from build123d import *

# Parameters (mm, degrees)
SKETCH1_R           = 2.5
BOSS_EXTRUDE1_DEPTH = 180


with BuildPart() as part:
    # Sketch1 → Boss-Extrude1 (new body)
    with BuildSketch(Plane.XY):
        with BuildLine():
            Line((2.839339828, 3.9), (5.5, 6.560660172))
            Line((5.5, 6.560660172), (5.5, 8.2))
            Line((5.5, 8.2), (3.1, 8.2))
            Line((3.1, 8.2), (3.1, 9.5))
            Line((3.1, 9.5), (3.6, 9.5))
            Line((3.6, 9.5), (3.6, 10))
            Line((3.6, 10), (8.5, 10))
            ThreePointArc((8.5, 10), (9.560660172, 9.560660172), (10, 8.5))
            Line((10, 8.5), (10, 3.6))
            Line((10, 3.6), (9.5, 3.6))
            Line((9.5, 3.6), (9.5, 3.1))
            Line((9.5, 3.1), (8.2, 3.1))
            Line((8.2, 3.1), (8.2, 5.5))
            Line((8.2, 5.5), (6.560660172, 5.5))
            Line((6.560660172, 5.5), (3.9, 2.839339828))
            Line((3.9, 2.839339828), (3.9, -2.839339828))
            Line((3.9, -2.839339828), (6.560660172, -5.5))
            Line((6.560660172, -5.5), (8.2, -5.5))
            Line((8.2, -5.5), (8.2, -3.1))
            Line((8.2, -3.1), (9.5, -3.1))
            Line((9.5, -3.1), (9.5, -3.6))
            Line((9.5, -3.6), (10, -3.6))
            Line((10, -3.6), (10, -8.5))
            ThreePointArc((10, -8.5), (9.560660172, -9.560660172), (8.5, -10))
            Line((8.5, -10), (3.6, -10))
            Line((3.6, -10), (3.6, -9.5))
            Line((3.6, -9.5), (3.1, -9.5))
            Line((3.1, -9.5), (3.1, -8.2))
            Line((3.1, -8.2), (5.5, -8.2))
            Line((5.5, -8.2), (5.5, -6.560660172))
            Line((5.5, -6.560660172), (2.839339828, -3.9))
            Line((2.839339828, -3.9), (-2.839339828, -3.9))
            Line((-2.839339828, -3.9), (-5.5, -6.560660172))
            Line((-5.5, -6.560660172), (-5.5, -8.2))
            Line((-5.5, -8.2), (-3.1, -8.2))
            Line((-3.1, -8.2), (-3.1, -9.5))
            Line((-3.1, -9.5), (-3.6, -9.5))
            Line((-3.6, -9.5), (-3.6, -10))
            Line((-3.6, -10), (-8.5, -10))
            ThreePointArc((-8.5, -10), (-9.560660172, -9.560660172), (-10, -8.5))
            Line((-10, -8.5), (-10, -3.6))
            Line((-10, -3.6), (-9.5, -3.6))
            Line((-9.5, -3.6), (-9.5, -3.1))
            Line((-9.5, -3.1), (-8.2, -3.1))
            Line((-8.2, -3.1), (-8.2, -5.5))
            Line((-8.2, -5.5), (-6.560660172, -5.5))
            Line((-6.560660172, -5.5), (-3.9, -2.839339828))
            Line((-3.9, -2.839339828), (-3.9, 2.839339828))
            Line((-3.9, 2.839339828), (-6.560660172, 5.5))
            Line((-6.560660172, 5.5), (-8.2, 5.5))
            Line((-8.2, 5.5), (-8.2, 3.1))
            Line((-8.2, 3.1), (-9.5, 3.1))
            Line((-9.5, 3.1), (-9.5, 3.6))
            Line((-9.5, 3.6), (-10, 3.6))
            Line((-10, 3.6), (-10, 8.5))
            ThreePointArc((-10, 8.5), (-9.560660172, 9.560660172), (-8.5, 10))
            Line((-8.5, 10), (-3.6, 10))
            Line((-3.6, 10), (-3.6, 9.5))
            Line((-3.6, 9.5), (-3.1, 9.5))
            Line((-3.1, 9.5), (-3.1, 8.2))
            Line((-3.1, 8.2), (-5.5, 8.2))
            Line((-5.5, 8.2), (-5.5, 6.560660172))
            Line((-5.5, 6.560660172), (-2.839339828, 3.9))
            Line((-2.839339828, 3.9), (2.839339828, 3.9))
        make_face()
        with Locations(Location((0, 0.235847297, 0), (0, 0, 180))):
            Circle(SKETCH1_R, mode=Mode.SUBTRACT)
    extrude(amount=BOSS_EXTRUDE1_DEPTH)


solid = part.part
The listing builds one solid part. Answer for the finished solid, in the listing's coordinates (mm). A direction names the side the tool comes from. Give positions to 0.01 mm unless a question says otherwise; leave off trailing zeros. Write each loop counter-clockwise with the first axis right and the second up, starting at its lowest first coordinate (ties: lowest second). Pieces come first, ordered by that corner, then holes.
Item 1: Which of the six approach directions +Z, -Z, +X, -X, +Y, -Y give full straight-line access (tool end or side, diameter ignored) to faces 4 (the flat face through (-3.9, 0, 89)), 5 (the flat face through (0, 3.9, 89)), 6 (the flat face through (3.9, 0, 89))?
Item 2: Determine the mould class of faces 1 (the flat face through (0, -3.9, 89)), 2 (the flat face through (-10, -6, 89)), 3 (the flat face through (6, -10, 89)) for opening direction X: released by +X, released by -X, zero draft, split by the parting line, or undercut.
Item 3: Find the intervals of material crossed by line 1 along X through (y, z) = (8.75, 139); line 2 along Y through (x, z) = (7.25, 21), in increasing order.
Item 4: Section A-A, the plane x = 0 is taken. Write down the section's boundary in (y, z), plus the area to 3 significant figures.
Item 5: Flat-ended cylindrical pins translate along their axes: P1, Ø4, axis at x = 0, y = 0.24, coming from the -Z side; P2, Ø0.6, axis at x = 10, z = 134, coming from the -Y side; P3, Ø1, axis at x = -3, z = 98, coming from the -Y side. Find the tip coordinate at first contact, or state that the pin passes through.
Completed:
1. face 4: +Z, -Z, -X
1. face 5: +Z, -Z, +Y
1. face 6: +Z, -Z, +X
2. face 1: undercut
2. face 2: released by -X
2. face 3: zero draft
3. line 1: x = -9.98 to -3.1, 3.1 to 9.98
3. line 2: y = -10 to -5.5, 5.5 to 10
4. outline: (-3.9, 0) - (-2.26, 0) - (-2.26, 180) - (-3.9, 180) - close; (2.74, 0) - (3.9, 0) - (3.9, 180) - (2.74, 180) - close
4. area: 504 mm2
5. P1: passes through
5. P2: stops at y = -9.4
5. P3: stops at y = -9.5
